```python
from build123d import *

# Parameters (mm, degrees)
F0_W      = 106.5
F0_H      = 72
F1_DEPTH  = 2.75
F2_W      = 98.5
F2_H      = 62.75
F2_H_2    = 1.25
F3_DEPTH  = 1.25
F4_W      = 8
F4_H      = 8
F5_DEPTH  = 12
F6_W      = 5
F6_H      = 8
F7_DEPTH  = 8
F11_D     = 3.25
F11_DEPTH = 8
F12_D     = 3.25
F12_DEPTH = 8
F13_D     = 3.25
F13_DEPTH = 8
F15_DEPTH = 2.5
F17_DEPTH = 1.75
F19_DEPTH = 1.75
F21_DEPTH = 2.5
F23_DEPTH = 1.75
F25_DEPTH = 1.75
F26_R     = 3


with BuildPart() as f1:
    # F0 (on Top) → F1 (new body)
    with BuildSketch(Plane.XY):
        Rectangle(F0_W, F0_H)
    extrude(amount=F1_DEPTH)

    # F2 (on face) → F3 (join)
    with BuildSketch(Plane.XY.offset(2.75)):
        with Locations((0, 0.625)):
            Rectangle(F2_W, F2_H)
        with Locations((0, -35.375)):
            Rectangle(F2_W, F2_H_2)
    extrude(amount=F3_DEPTH)

    # F4 (on face) → F5 (join)
    with BuildSketch(Plane.XY.offset(4)):
        with Locations((-45.25, 28)):
            Rectangle(F4_W, F4_H)
        with Locations((45.25, 28)):
            Rectangle(F4_W, F4_H)
    extrude(amount=F5_DEPTH)

    # F6 (on face) → F7 (join)
    with BuildSketch(Plane.XY.offset(4)):
        with Locations((-46.75, -14)):
            Rectangle(F6_W, F6_H)
        with Locations((46.75, -14)):
            Rectangle(F6_W, F6_H)
    extrude(amount=F7_DEPTH)

    # F11
    with Locations(Plane(origin=(0, 32, 0), x_dir=(-1, 0, 0), z_dir=(0, 1, 0))):
        with Locations((-45.303469, 12), (45.25, 12)):
            Hole(F11_D / 2, depth=F11_DEPTH)

    # F12
    with Locations(Plane(origin=(-49.25, 0, 0), x_dir=(0, -1, 0), z_dir=(-1, 0, 0))):
        with Locations((-28, 8), (14, 8)):
            Hole(F12_D / 2, depth=F12_DEPTH)

    # F13
    with Locations(Plane.YZ.offset(49.25)):
        with Locations((-14, 8), (28, 8)):
            Hole(F13_D / 2, depth=F13_DEPTH)

    # F14 (on face) → F15 (cut)
    with BuildSketch(Plane.YZ.offset(-44.25)):
        Polygon((-11.125, 6.340118), (-11.125, 9.659882), (-14, 11.319764), (-16.875, 9.659882), (-16.875, 6.340118), (-14, 4.680236), align=None)
    extrude(amount=-F15_DEPTH, mode=Mode.SUBTRACT)

    # F16 (on face) → F17 (cut)
    with BuildSketch(Plane.YZ.offset(-41.25)):
        Polygon((30.844677, 9.711329), (27.940285, 11.319227), (25.095607, 9.607898), (25.155323, 6.288671), (28.059715, 4.680773), (30.904393, 6.392102), align=None)
    extrude(amount=-F17_DEPTH, mode=Mode.SUBTRACT)

    # F18 (on face) → F19 (cut)
    with BuildSketch(Plane(origin=(41.25, 0, 0), x_dir=(0, -1, 0), z_dir=(-1, 0, 0))):
        Polygon((-25.109566, 9.632858), (-27.968879, 11.319618), (-30.859313, 9.68676), (-30.890434, 6.367142), (-28.031121, 4.680382), (-25.140687, 6.31324), align=None)
    extrude(amount=-F19_DEPTH, mode=Mode.SUBTRACT)

    # F20 (on face) → F21 (cut)
    with BuildSketch(Plane(origin=(44.25, 0, 0), x_dir=(0, -1, 0), z_dir=(-1, 0, 0))):
        Polygon((13.950525, 11.319395), (11.100582, 9.616851), (11.150057, 6.297455), (14.049475, 4.680605), (16.899418, 6.383149), (16.849943, 9.702545), align=None)
    extrude(amount=-F21_DEPTH, mode=Mode.SUBTRACT)

    # F22 (on face) → F23 (cut)
    with BuildSketch(Plane.XZ.offset(-24)):
        Polygon((-42.375, 10.340118), (-42.375, 13.659882), (-45.25, 15.319764), (-48.125, 13.659882), (-48.125, 10.340118), (-45.25, 8.680236), align=None)
    extrude(amount=-F23_DEPTH, mode=Mode.SUBTRACT)

    # F24 (on face) → F25 (cut)
    with BuildSketch(Plane.XZ.offset(-24)):
        Polygon((41.983721, 12.010152), (43.634803, 9.130089), (46.954552, 9.119938), (48.623218, 11.989848), (46.972135, 14.869911), (43.652387, 14.880062), align=None)
    extrude(amount=-F25_DEPTH, mode=Mode.SUBTRACT)

    # F26
    f26_edges = [f1.edges().sort_by_distance(p)[0] for p in [
        (46.75, -18, 12),
        (46.75, -10, 12),
        (-46.75, -18, 12),
        (-46.75, -10, 12),
        (-41.25, 28, 16),
        (41.25, 28, 16),
    ]]
    fillet(f26_edges, radius=F26_R)


solid = f1.part
```
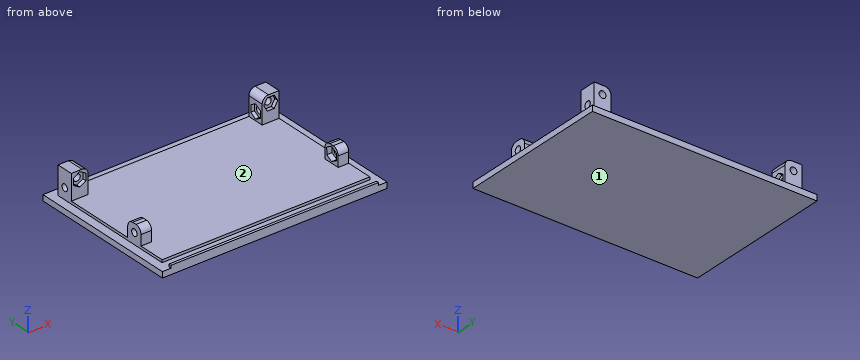
Model file for the job. Use its own axes, mm. Face numbers are marked on the shaded views. Give positions to 0.01 mm unless a question says otherwise; leave off trailing zeros. Write each loop counter-clockwise with the first axis right and the second up, starting at its lowest first coordinate (ties: lowest second). Pieces come first, ordered by that corner, then holes. Notation, with made-up numbers: M 41.5,-19 L 82.5,-19 A31 cw 82.5,8 Z; hole C 77,-16 d10. An arc over 180 degrees is marked long. Use a Markdown table: item, result.
1) Pull direction X, two halves, no side cores. Call the marked faces 1 and 2: +X half, -X half, draft (parallel to the pull), parting line (faces both ways), or undercut.
Responses:
| item | result |
|---|---|
| face 1 | draft |
| face 2 | undercut |
2) Cut at B-B (y = 17). List the corners of the cut face in (x, z), and give its area (3 significant figures).
Responses:
| item | result |
|---|---|
| outline | M -53.25,0 L 53.25,0 L 53.25,2.75 L 49.25,2.75 L 49.25,4 L -49.25,4 L -49.25,2.75 L -53.25,2.75 Z |
| area | 416 mm2 |
3) Pin check, flat tips, straight feed: pin 1 (2 mm diameter, centred on x = -0.5, y = 0, fed in from -Z); pin 2 (1 mm diameter, centred on x = 2.5, y = 9.5, fed in from +Z); pin 3 (4.5 mm diameter, centred on y = -14.5, z = 8, fed in from +X); pin 4 (0.6 mm diameter, centred on x = -18.5, z = 3.5, fed in from +Y). Stop position of each tip, or through.
Responses:
| item | result |
|---|---|
| pin 1 | stops at z = 0 |
| pin 2 | stops at z = 4 |
| pin 3 | stops at x = 49.25 |
| pin 4 | stops at y = 32 |
4) Cut at A-A (x = 4). List the corners of the cut face in (y, z), and give its area (3 significant figures).
Responses:
| item | result |
|---|---|
| outline | M -36,0 L 36,0 L 36,2.75 L 32,2.75 L 32,4 L -30.75,4 L -30.75,2.75 L -34.75,2.75 L -34.75,4 L -36,4 Z |
| area | 278 mm2 |
5) Drill centre lines: line 1 (Z direction, x = -47.3, y = -14) (3 decimals); line 2 (Z direction, x = 45.5, y = 30); line 3 (Z direction, x = -5.5, y = 30.5). Where is each one in solid material? Low to high. Write a range as from..to.
Responses:
| item | result |
|---|---|
| line 1 | z = 0..6.375, 9.625..12 |
| line 2 | z = 0..10.39, 13.61..16 |
| line 3 | z = 0..4 |
